Design review of the part shown in the three views and the two pictorial views. Dimensions are in mm from the part's minimum x, y and z. A direction names the side the tool comes from. Coordinates: 2 decimals unless noted, no trailing zeros. Write each loop counter-clockwise with the first axis right and the second up, starting at its lowest first coordinate (ties: lowest second). Pieces come first, ordered by that corner, then holes. Notation, with made-up numbers: (29, 24) -> (56, 24) arc R15 ccw to (56, 39) -> close; hole circle Ø1 at (21.25, 45.25). An arc over 180 degrees is marked (long way). Answer in a Markdown table with one row per item. Add a question column.
Item 1: For the marked faces 4 and 5, list the 3-axis set-ups (+Z, -Z, +X, -X, +Y, -Y) from which the entire face can be reached by the end or side of a thin tool; tool diameter is ignored.
Item 2: Take a section at B-B, the plane x = 1.5. Write out the cut boundary in (y, z), and give its area (3 significant figures).
Item 3: Draft analysis for pull direction X (two halves, no side actions). For the marked faces 1, 2 and 3, state which applies: released by +X, released by -X, zero draft, split by the parting line, or undercut.
Item 4: To check wall thickness, follow line 1 (Y direction, x = 4, z = 19.75); line 2 (Y direction, x = 4, z = 2.75); line 3 (Z direction, x = 4.5, y = 7). State the ranges of each line that lie inside material, in increasing order.
Item 5: Take a section at D-D, the plane z = 9.25. Write out the cut boundary in (x, y).
Item 6: Take a section at A-A, the plane z = 5. Write out the cut boundary in (x, y).
Item 7: Take a section at C-C, the plane y = 1.75. Write out the cut boundary in (x, z).
Item 8: Clearance check with flat-ended pins moving along their axes: P1, Ø1.5, axis at y = 5, z = 7, coming from the -X side; P2, Ø2, axis at x = 4, y = 4, coming from the -Z side; P3, Ø3, axis at x = 5.5, z = 17, coming from the -Y side (1 decimal). State where each tip first meets the part, or that it passes through.
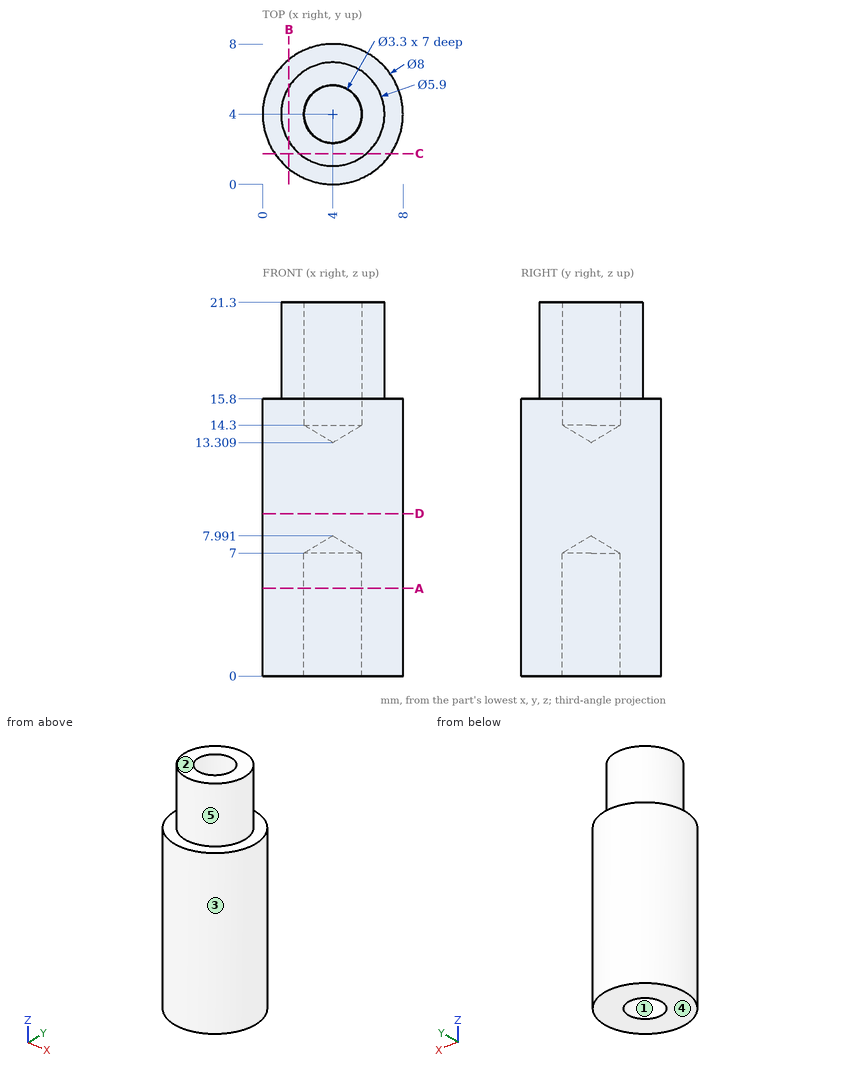
Answers:
| question | item | result |
|---|---|---|
| 1 | face 4 | -Z, +X, -X, +Y, -Y |
| 1 | face 5 | +Z |
| 2 | outline | (0.88, 0) -> (7.12, 0) -> (7.12, 15.8) -> (5.57, 15.8) -> (5.57, 21.3) -> (2.43, 21.3) -> (2.43, 15.8) -> (0.88, 15.8) -> close |
| 2 | area | 116 mm^2 |
| 3 | face 1 | undercut |
| 3 | face 2 | zero draft |
| 3 | face 3 | split by the parting line |
| 4 | line 1 | y = 1.05 to 2.35, 5.65 to 6.95 |
| 4 | line 2 | y = 0 to 2.35, 5.65 to 8 |
| 4 | line 3 | z = 0 to 15.8 |
| 5 | outline | circle Ø8 at (4, 4) |
| 6 | outline | circle Ø8 at (4, 4); hole circle Ø3.3 at (4, 4) |
| 7 | outline | (0.69, 0) -> (7.31, 0) -> (7.31, 15.8) -> (5.91, 15.8) -> (5.91, 21.3) -> (2.09, 21.3) -> (2.09, 15.8) -> (0.69, 15.8) -> close |
| 8 | P1 | stops at x = 0.01 |
| 8 | P2 | stops at z = 7.39 |
| 8 | P3 | stops at y = 0 |
